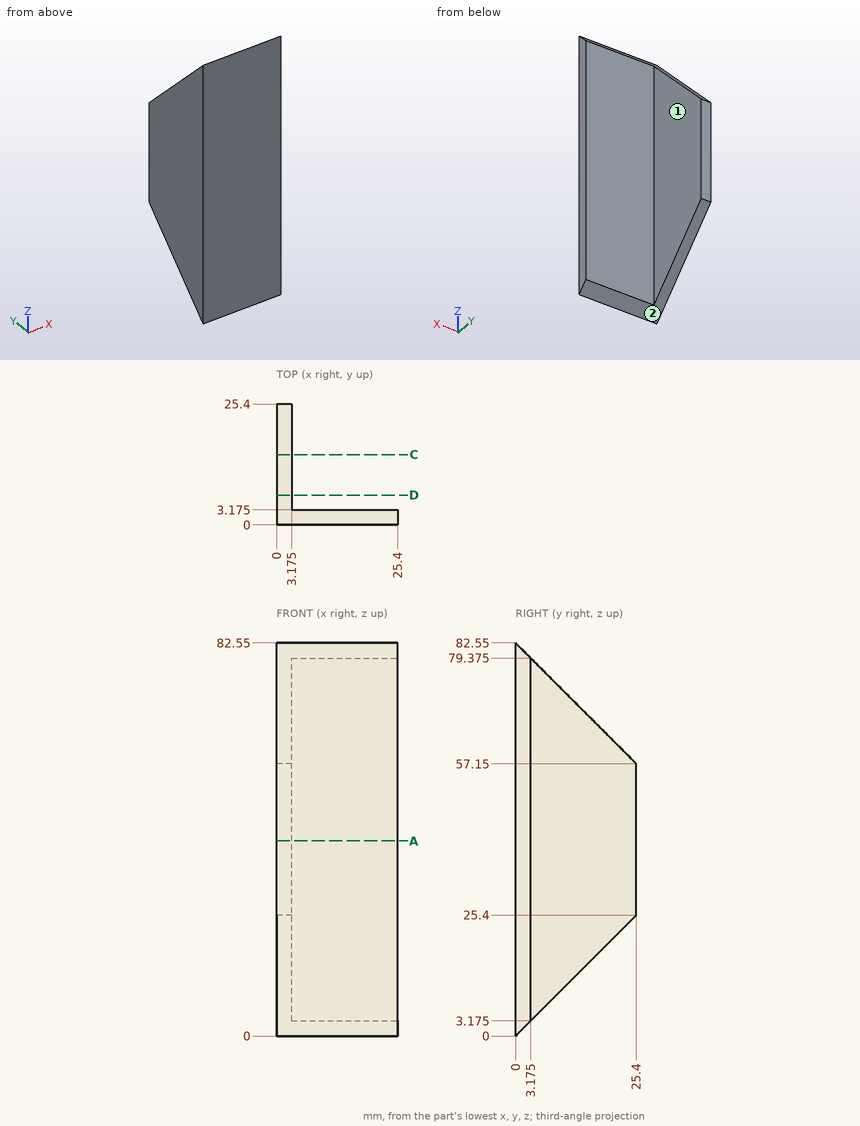
Verification items for this drawing (mm, ordinates from the low corner). A direction names the side the tool comes from. Give positions to 0.01 mm unless a question says otherwise; leave off trailing zeros. Write each loop counter-clockwise with the first axis right and the second up, starting at its lowest first coordinate (ties: lowest second). Pieces come first, ordered by that corner, then holes. Notation, with made-up numbers: (-39, 20) - (5, 20) arc R21 ccw to (5, 31) - close; hole circle Ø5 at (-9.5, 46). An arc over 180 degrees is marked (long way). Answer as a JSON object with one key per item and string values. Group by question number.
1) Sectioned sample at A-A (z = 41). Record the cut outline in (x, y) (3 decimals), then the cut area to 3 significant figures.
2) Thickness scan on probe 1 along Y at (x, z) = (22.25, 63.5) (3 decimals); probe 2 along Z at (x, y) = (14, 2). Record the ranges inside material, lowest first. Write a range as from..to.
3) Sectioned sample at D-D (y = 6.25). Record the cut outline in (x, z) (3 decimals), then the cut area to 3 significant figures.
4) Access from +Z, -Z, +X, -X, +Y, -Y to the whole of each face (thin tool, end or side, straight path). Record for the marked faces 1 and 2.
5) Sectioned sample at C-C (y = 14.75). Record the cut outline in (x, z) (3 decimals), then the cut area to 3 significant figures.
6) Depth check by flat-ended pin: P1, Ø5, axis at x = 9, z = 46.5, coming from the +Y side (3 decimals); P2, Ø1, axis at x = 14, y = 3, coming from the -Z side; P3, Ø8, axis at y = 21.5, z = 62, coming from the +X side (3 decimals). Enter the tip coordinate at first touch or a pass-through.
Geometry results:
{
 "1": {"outline": "(0, 0) - (25.4, 0) - (25.4, 3.175) - (3.175, 3.175) - (3.175, 25.4) - (0, 25.4) - close", "area": "151 mm^2"},
 "2": {"probe 1": "y = 0..3.175", "probe 2": "z = 2..80.55"},
 "3": {"outline": "(0, 6.25) - (3.175, 6.25) - (3.175, 76.3) - (0, 76.3) - close", "area": "222 mm^2"},
 "4": {"face 1": "+Z, -Z, +X, +Y", "face 2": "-Z, +X, -X, +Y"},
 "5": {"outline": "(0, 14.75) - (3.175, 14.75) - (3.175, 67.8) - (0, 67.8) - close", "area": "168 mm^2"},
 "6": {"P1": "stops at y = 3.175", "P2": "stops at z = 2.5", "P3": "stops at x = 3.175"}
}
